```python
from build123d import *

# Parameters (mm, degrees)
F1_DEPTH = 558.8
F2_W     = 12.7
F2_H     = 5.08
F3_DEPTH = 2.38125
F4_DEPTH = 2.38125
F5_W     = 12.7
F5_H     = 5.08
F6_DEPTH = 2.38125
F8_DEPTH = 533.4
F9_DEPTH = 82.55


with BuildPart() as f1:
    # F0 (on Right) → F1 (new body)
    with BuildSketch(Plane.YZ):
        with BuildLine():
            Line((73.152, 0), (3.048, 0))
            ThreePointArc((3.048, 0), (0.892739, -0.892739), (0, -3.048))
            Line((0, -3.048), (0, -73.152))
            ThreePointArc((0, -73.152), (0.892739, -75.307261), (3.048, -76.2))
            Line((3.048, -76.2), (73.152, -76.2))
            ThreePointArc((73.152, -76.2), (75.307261, -75.307261), (76.2, -73.152))
            Line((76.2, -73.152), (76.2, -3.048))
            ThreePointArc((76.2, -3.048), (75.307261, -0.892739), (73.152, 0))
        make_face()
        with BuildLine():
            ThreePointArc((73.152, -2.38125), (73.623463, -2.576537), (73.81875, -3.048))
            Line((73.81875, -3.048), (73.81875, -73.152))
            ThreePointArc((73.81875, -73.152), (73.623463, -73.623463), (73.152, -73.81875))
            Line((73.152, -73.81875), (3.048, -73.81875))
            ThreePointArc((3.048, -73.81875), (2.576537, -73.623463), (2.38125, -73.152))
            Line((2.38125, -73.152), (2.38125, -3.048))
            ThreePointArc((2.38125, -3.048), (2.576537, -2.576537), (3.048, -2.38125))
            Line((3.048, -2.38125), (73.152, -2.38125))
        make_face(mode=Mode.SUBTRACT)
    extrude(amount=F1_DEPTH)

    # F2 (on face) → F3 (cut)
    with BuildSketch(Plane.XY):
        with Locations((473.075, 60.96)):
            Rectangle(F2_W, F2_H)
        with Locations((473.075, 15.24)):
            Rectangle(F2_W, F2_H)
        with Locations((406.527, 15.24)):
            Rectangle(F2_W, F2_H)
        with Locations((406.527, 60.96)):
            Rectangle(F2_W, F2_H)
    extrude(amount=-F3_DEPTH, mode=Mode.SUBTRACT)

    # F2 (on face) → F4 (cut)
    with BuildSketch(Plane.XY):
        with Locations((168.275, 60.96)):
            Rectangle(F2_W, F2_H)
        with Locations((168.275, 15.24)):
            Rectangle(F2_W, F2_H)
        with Locations((101.727, 15.24)):
            Rectangle(F2_W, F2_H)
        with Locations((101.727, 60.96)):
            Rectangle(F2_W, F2_H)
    extrude(amount=-F4_DEPTH, mode=Mode.SUBTRACT)

    # F5 (on face) → F6 (cut)
    with BuildSketch(Plane.XZ):
        with Locations((473.075, -15.24)):
            Rectangle(F5_W, F5_H)
        with Locations((473.075, -60.96)):
            Rectangle(F5_W, F5_H)
        with Locations((406.527, -60.96)):
            Rectangle(F5_W, F5_H)
        with Locations((406.527, -15.24)):
            Rectangle(F5_W, F5_H)
        with Locations((168.275, -60.96)):
            Rectangle(F5_W, F5_H)
        with Locations((168.275, -15.24)):
            Rectangle(F5_W, F5_H)
        with Locations((101.727, -60.96)):
            Rectangle(F5_W, F5_H)
        with Locations((101.727, -15.24)):
            Rectangle(F5_W, F5_H)
    extrude(amount=-F6_DEPTH, mode=Mode.SUBTRACT)

    # F7 (on face) → F8 (join)
    with BuildSketch(Plane.YZ.offset(558.8)):
        Polygon((88.9, -27.94), (76.2, -27.94), (76.2, -40.64), (79.375, -40.64), (79.375, -31.115), (88.9, -31.115), align=None)
        Polygon((40.64, -79.375), (40.64, -76.2), (27.94, -76.2), (27.94, -88.9), (31.115, -88.9), (31.115, -79.375), align=None)
    extrude(amount=-F8_DEPTH)

    # F7 (on face) → F9 (cut)
    with BuildSketch(Plane.YZ.offset(558.8)):
        Polygon((88.9, -27.94), (76.2, -27.94), (76.2, -40.64), (79.375, -40.64), (79.375, -31.115), (88.9, -31.115), align=None)
        Polygon((40.64, -79.375), (40.64, -76.2), (27.94, -76.2), (27.94, -88.9), (31.115, -88.9), (31.115, -79.375), align=None)
    extrude(amount=-F9_DEPTH, mode=Mode.SUBTRACT)


solid = f1.part
```
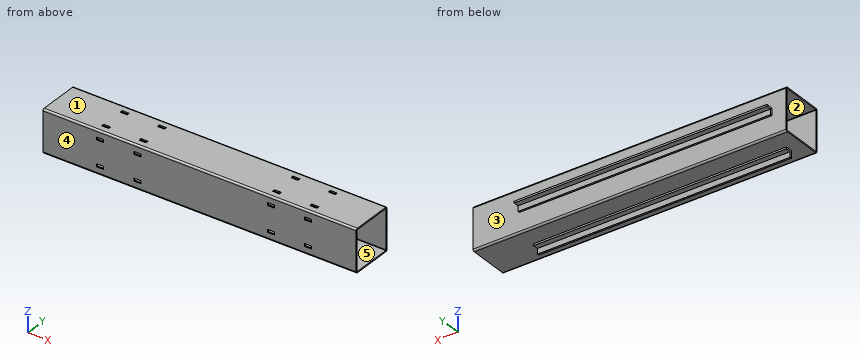
Here's how the part is built. I have some questions about the finished solid (model axes, mm). Face numbers are marked on the shaded views. A direction names the side the tool comes from. Coordinates: 2 decimals unless noted, no trailing zeros. Loops run counter-clockwise (first coordinate to the right, second up) from the corner with the lowest first, then second, coordinate; pieces in that order, holes last. Notation, with made-up numbers: (60.25, -20.75) -> (68.25, -20.75) arc R6 cw to (68.25, -9.75) -> close; hole circle Ø5 at (66, 20.25). An arc over 180 degrees is marked (long way). Return JSON: item names as keys, results as strings.
1) If we section it at C-C, the plane y = 48.5: Write out the boundary of the cut face in (x, z).
Results below:
{"outline": "(0, -76.2) -> (558.8, -76.2) -> (558.8, -73.82) -> (0, -73.82) -> close; (0, -2.38) -> (558.8, -2.38) -> (558.8, 0) -> (0, 0) -> close"}
2) If we section it at A-A, the plane z = -51: Write out the boundary of the cut face in (x, y).
Results below:
{"outline": "(0, 0) -> (558.8, 0) -> (558.8, 2.38) -> (0, 2.38) -> close; (0, 73.82) -> (558.8, 73.82) -> (558.8, 76.2) -> (0, 76.2) -> close"}
3) If we section it at B-B, the plane x = 88.5: Write out the boundary of the cut face in (y, z) (1 decimal), then the cut area to 3 significant figures.
Results below:
{"outline": "(0, -73.2) arc R3 ccw to (3, -76.2) -> (27.9, -76.2) -> (27.9, -88.9) -> (31.1, -88.9) -> (31.1, -79.4) -> (40.6, -79.4) -> (40.6, -76.2) -> (73.2, -76.2) arc R3 ccw to (76.2, -73.2) -> (76.2, -40.6) -> (79.4, -40.6) -> (79.4, -31.1) -> (88.9, -31.1) -> (88.9, -27.9) -> (76.2, -27.9) -> (76.2, -3) arc R3 ccw to (73.2, 0) -> (3, 0) arc R3 ccw to (0, -3) -> close; hole (2.4, -73.2) arc R0.7 ccw to (3, -73.8) -> (73.2, -73.8) arc R0.7 ccw to (73.8, -73.2) -> (73.8, -3) arc R0.7 ccw to (73.2, -2.4) -> (3, -2.4) arc R0.7 ccw to (2.4, -3) -> close", "area": "837 mm²"}
4) Will these pins go through, and if not, where does the flat tip stop? pin 1 (4 mm diameter, centred on x = 314, y = 76.5, fed in from +Z); pin 2 (2.5 mm diameter, centred on x = 403.5, z = -0.5, fed in from -Y); pin 3 (2.5 mm diameter, centred on x = 169, y = 1, fed in from -Z).
Results below:
{"pin 1": "z = -0.31", "pin 2": "y = 0.29", "pin 3": "z = -76.09"}
5) For the marked faces 4 and 5, which set-ups out of +Z, -Z, +X, -X, +Y, -Y let a thin tool reach every point of the face, with its end or its side?
Results below:
{"face 4": "+Z, -Z, +X, -X, -Y", "face 5": "+X, -X"}
6) Thinking about a two-plate mould opening in Z: for the marked faces 1, 2 and 3, which applies, +Z half, -Z half, draft (parallel to the pull), parting line (faces both ways), or undercut?
Results below:
{"face 1": "+Z half", "face 2": "undercut", "face 3": "draft"}
7) I need wall thicknesses on line 1 (Z direction, x = 251, y = 53); line 2 (Z direction, x = 64.5, y = 36.5) (3 decimals); line 3 (Y direction, x = 57.5, z = -25.5). Which ranges of each line are inside material? Lowest first, please. Write a range as from..to.
Results below:
{"line 1": "-76.2..-73.82, -2.38..0", "line 2": "-79.375..-73.819, -2.381..0", "line 3": "0..2.38, 73.82..76.2"}
